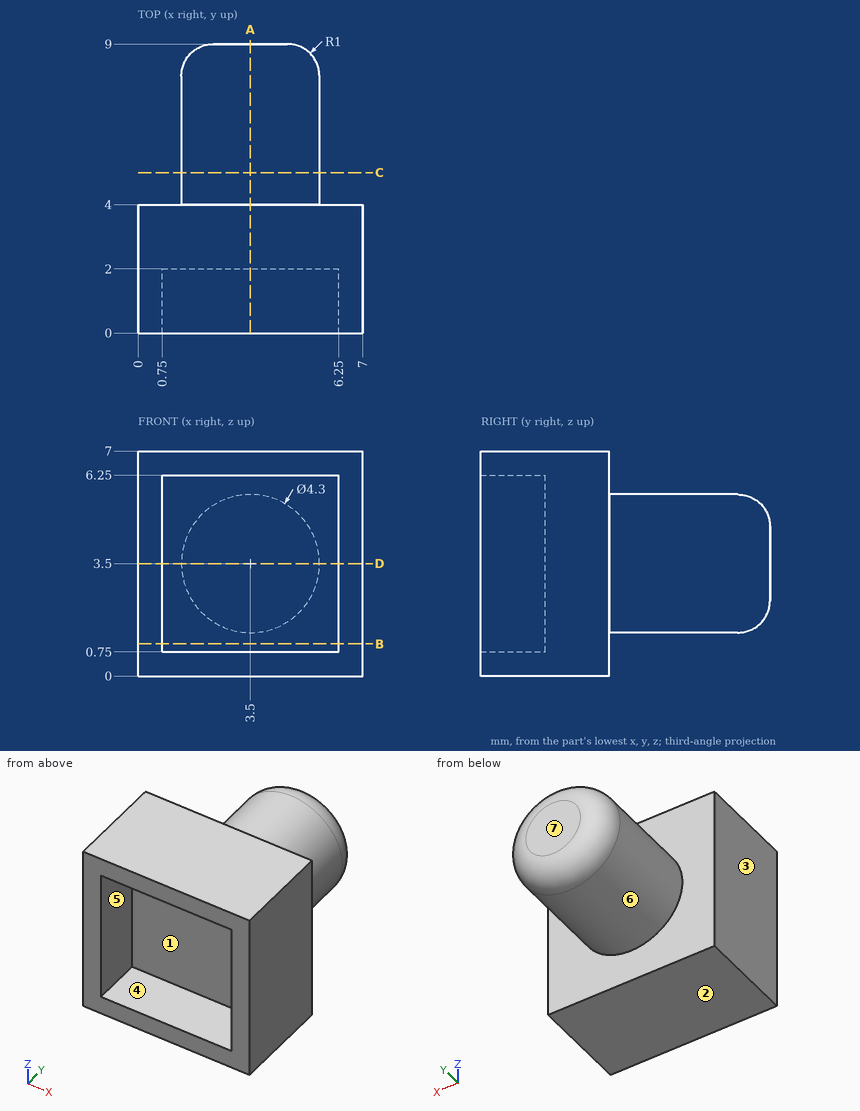
The drawing under review shows one solid part. Ordinate dimensions are in mm from its lowest x, y, z. A direction names the side the tool comes from. Coordinates: 2 decimals unless noted, no trailing zeros. Order: outer loops, then holes, each group sorted by start corner. A loop starts at its lowest first (then second) coordinate and runs counter-clockwise, first axis right, second up. Notation, with made-up numbers: (66, 85.25) -> (83, 85.25) arc R20 cw to (83, 123.25) -> close; hole circle Ø10 at (3.5, 51). An arc over 180 degrees is marked (long way). One line per item, written item: value.
1) We need section D-D, the plane z = 3.5. Give the boundary of the cut face in (x, y), then the cut area to 3 significant figures.
Output values:
outline: (0, 0) -> (0.75, 0) -> (0.75, 2) -> (6.25, 2) -> (6.25, 0) -> (7, 0) -> (7, 4) -> (5.65, 4) -> (5.65, 8) arc R1 ccw to (4.65, 9) -> (2.35, 9) arc R1 ccw to (1.35, 8) -> (1.35, 4) -> (0, 4) -> close
area: 38.1 mm2
2) We need section A-A, the plane x = 3.5. Give the boundary of the cut face in (y, z).
Output values:
outline: (0, 0) -> (4, 0) -> (4, 1.35) -> (8, 1.35) arc R1 ccw to (9, 2.35) -> (9, 4.65) arc R1 ccw to (8, 5.65) -> (4, 5.65) -> (4, 7) -> (0, 7) -> (0, 6.25) -> (2, 6.25) -> (2, 0.75) -> (0, 0.75) -> close
3) We need section C-C, the plane y = 5. Give the boundary of the cut face in (x, z), then the cut area to 3 significant figures.
Output values:
outline: circle Ø4.3 at (3.5, 3.5)
area: 14.5 mm2
4) To check wall thickness, follow probe 1 along Z at (x, y) = (4.75, 1.5); probe 2 along Y at (x, z) = (1.5, 6). State the ranges of each line that lie inside material, in increasing order. Write a range as [from, to].
Output values:
probe 1: z = [0, 0.75], [6.25, 7]
probe 2: y = [2, 4]
5) Machinability: for the marked faces 5, 6 and 7, which of the approach directions +Z, -Z, +X, -X, +Y, -Y give a long, thin tool a straight path to every point of the face, cutting with its end or side? Answer none if there is none.
Output values:
face 5: -Y
face 6: +Y
face 7: +Z, -Z, +X, -X, +Y
6) We need section B-B, the plane z = 1. Give the boundary of the cut face in (x, y), then the cut area to 3 significant figures.
Output values:
outline: (0, 0) -> (0.75, 0) -> (0.75, 2) -> (6.25, 2) -> (6.25, 0) -> (7, 0) -> (7, 4) -> (0, 4) -> close
area: 17.0 mm2
7) Clearance check with flat-ended pins moving along their axes: P1, Ø2, axis at y = 7.5, z = 2, coming from the +X side; P2, Ø1, axis at x = 2.5, z = 4, coming from the -Y side. State where each tip first meets the part, or that it passes through.
Output values:
P1: stops at x = 5.59
P2: stops at y = 2
8) Draft analysis for pull direction X (two halves, no side actions). For the marked faces 1, 2, 3 and 4, state which applies: +X half, -X half, draft (parallel to the pull), parting line (faces both ways), or undercut.
Output values:
face 1: undercut
face 2: draft
face 3: -X half
face 4: undercut
